Build history of the part. All positions in model axes, mm. A direction names the side the tool comes from. Coordinates: 2 decimals unless noted, no trailing zeros. Write each loop counter-clockwise with the first axis right and the second up, starting at its lowest first coordinate (ties: lowest second). Pieces come first, ordered by that corner, then holes. Notation, with made-up numbers: (88, 24) -> (141, 24) arc R33 cw to (141, 62) -> close; hole circle Ø10 at (5, -1). An arc over 180 degrees is marked (long way). Write each question's results on one line, items separated by ' | '. Start each with the question number.
Q1. Saw through at B-B on z = 32.5. Give the cut face in (x, y), and give its area (3 significant figures).
Q2. Tool access for faces 4 (the face through (6, 4, 26.303)), 5 (the face through (40, 5, -23.097)), 6 (the face through (-7.56, 11.65, -4.66)): list every direction of +Z, -Z, +X, -X, +Y, -Y with a clear straight run to the whole face (end or side of a thin tool).
Q3. Saw through at C-C on x = -15.5. Give the cut face in (y, z), and give its area (3 significant figures).
Q4. Saw through at A-A on z = 15.5. Give the cut face in (x, y), and give its area (3 significant figures).
Q5. Saw through at D-D on y = 13. Give the cut face in (x, z) (3 decimals), and give its area (3 significant figures).
Q6. Drop flat-ended pins along their axis: pin 1 Ø1 at (x, z) = (18, -14) entering from +Y; pin 2 Ø1 at (x, z) = (13, 28) entering from +Y; pin 3 Ø1.3 at (x, y) = (-6, 9) entering from -Z; pin 4 Ø5 at (y, z) = (9, -2) entering from -X. Give the stop position or say it passes through.
Q7. Drill centre lines: line 1 (X direction, y = 3, z = 11); line 2 (Y direction, x = 69, z = -8.5); line 3 (Y direction, x = 6.5, z = 4.5). Where is each one in solid material? Low to high.
Q8. Two-plate mould, pull along Z, no slides. Class faces 1 (the face through (-7, 15, 24)), 2 (the face through (4.412, 8, 29)), 3 (the face through (107.31, 5.03, -22.24)): released by +Z, released by -Z, zero draft, split by the parting line, or undercut.
from build123d import *

# Parameters (mm, degrees)
SKETCH1_W           = 134
SKETCH1_H           = 67
BOSS_EXTRUDE1_DEPTH = 10
SKETCH2_W           = 19.1
SKETCH2_H           = 19.1
CUT_EXTRUDE1_DEPTH  = 10
SKETCH2_3_R         = 1.275
BOSS_EXTRUDE2_DEPTH = 5
CUT_EXTRUDE3_START  = -1.6
SKETCH2_6_R         = 1.275
CUT_EXTRUDE3_DEPTH  = 1.6
SKETCH2_5_W         = 3.9
SKETCH2_5_H         = 3.1
SKETCH2_5_H_2       = 0.9
CUT_EXTRUDE2_DEPTH  = 3.14
FILLET1_R           = 3
FILLET2_R           = 1.5
FILLET3_R           = 1.5


with BuildPart() as part:
    # Sketch1 → Boss-Extrude1 (new body)
    with BuildSketch(Plane(origin=(0, 0, 0), x_dir=(1, 0, 0), z_dir=(0, 1, 0))):
        with Locations((41.212068984, -10.4030388)):
            Rectangle(SKETCH1_W, SKETCH1_H)
    extrude(amount=BOSS_EXTRUDE1_DEPTH)

    # Sketch2 → Cut-Extrude1 (cut)
    with BuildSketch(Plane(origin=(0, 10, 0), x_dir=(1, 0, 0), z_dir=(0, 1, 0))):
        with Locations((6.362068984, -16.7530388)):
            Rectangle(SKETCH2_W, SKETCH2_H)
    extrude(amount=-CUT_EXTRUDE1_DEPTH, mode=Mode.SUBTRACT)

    # Sketch2<3> → Boss-Extrude2 (add)
    with BuildSketch(Plane(origin=(0, 10, 0), x_dir=(1, 0, 0), z_dir=(0, 1, 0))):
        with Locations(Location((-6.787931016, 3.6469612, 0), (0, 0, 270))):
            Circle(SKETCH2_3_R)
        with Locations(Location((-6.787931016, -24.4530388, 0), (0, 0, 270))):
            Circle(SKETCH2_3_R)
        with Locations(Location((21.212068984, -24.4530388, 0), (0, 0, 270))):
            Circle(SKETCH2_3_R)
        with Locations(Location((21.212068984, 3.6469612, 0), (0, 0, 270))):
            Circle(SKETCH2_3_R)
    extrude(amount=BOSS_EXTRUDE2_DEPTH)

    # Sketch2<6> → Cut-Extrude3 (cut)
    with BuildSketch(Plane(origin=(0, 10, 0), x_dir=(1, 0, 0), z_dir=(0, 1, 0)).offset(CUT_EXTRUDE3_START)):
        Polygon((26.212068984, 8.5969612), (-11.787931016, 8.5969612), (-11.787931016, -29.4030388), (4.412068984, -29.4030388), (4.412068984, -26.3030388), (-3.187931016, -26.3030388), (-3.187931016, -7.2030388), (15.912068984, -7.2030388), (15.912068984, -26.3030388), (8.312068984, -26.3030388), (8.312068984, -29.4030388), (26.212068984, -29.4030388), align=None)
        with Locations(Location((-6.787931016, -24.4530388, 0), (0, 0, 270))):
            Circle(SKETCH2_6_R, mode=Mode.SUBTRACT)
        with Locations(Location((21.212068984, -24.4530388, 0), (0, 0, 270))):
            Circle(SKETCH2_6_R, mode=Mode.SUBTRACT)
        with Locations(Location((-6.787931016, 3.6469612, 0), (0, 0, 270))):
            Circle(SKETCH2_6_R, mode=Mode.SUBTRACT)
        with Locations(Location((21.212068984, 3.6469612, 0), (0, 0, 270))):
            Circle(SKETCH2_6_R, mode=Mode.SUBTRACT)
    extrude(amount=CUT_EXTRUDE3_DEPTH, mode=Mode.SUBTRACT)

    # Sketch2<5> → Cut-Extrude2 (cut)
    with BuildSketch(Plane(origin=(0, 10, 0), x_dir=(1, 0, 0), z_dir=(0, 1, 0))):
        with Locations((6.362068984, -27.8530388)):
            Rectangle(SKETCH2_5_W, SKETCH2_5_H)
        with Locations((6.362068984, -29.8530388)):
            Rectangle(SKETCH2_5_W, SKETCH2_5_H_2)
    extrude(amount=-CUT_EXTRUDE2_DEPTH, mode=Mode.SUBTRACT)

    # Fillet1
    fillet1_edges = [part.edges().sort_by_distance(p)[0] for p in [
        (108.212068984, 10, 10.4030388),
        (41.212068984, 10, -23.0969612),
        (-25.787931016, 10, 10.4030388),
        (41.212068984, 0, -23.0969612),
        (108.212068984, 0, 10.4030388),
        (41.212068984, 0, 43.9030388),
        (-25.787931016, 0, 10.4030388),
        (-25.787931016, 5, -23.0969612),
        (108.212068984, 5, -23.0969612),
        (108.212068984, 5, 43.9030388),
        (-25.787931016, 5, 43.9030388),
        (41.212068984, 10, 43.9030388),
    ]]
    fillet(fillet1_edges, radius=FILLET1_R)

    # Fillet2
    fillet2_edges = [part.edges().sort_by_distance(p)[0] for p in [
        (4.412068984, 7.63, 26.3030388),
        (6.362068984, 6.86, 26.3030388),
        (-3.187931016, 4.2, 26.3030388),
        (15.912068984, 4.2, 26.3030388),
        (15.912068984, 0, 16.7530388),
        (6.362068984, 0, 26.3030388),
        (-3.187931016, 0, 16.7530388),
        (15.912068984, 8.4, 16.7530388),
        (6.362068984, 8.4, 7.2030388),
        (12.112068984, 8.4, 26.3030388),
        (-3.187931016, 8.4, 16.7530388),
        (0.612068984, 8.4, 26.3030388),
        (8.312068984, 7.63, 26.3030388),
    ]]
    fillet(fillet2_edges, radius=FILLET2_R)

    # Fillet3
    fillet3_edges = [part.edges().sort_by_distance(p)[0] for p in [
        (7.212068984, 10, -8.5969612),
        (26.212068984, 10, 10.4030388),
        (-11.787931016, 10, 10.4030388),
    ]]
    fillet(fillet3_edges, radius=FILLET3_R)


solid = part.part
Returned:
1) outline: (-25.79, 3) arc R3 ccw to (-22.79, 0) -> (105.21, 0) arc R3 ccw to (108.21, 3) -> (108.21, 7) arc R3 ccw to (105.21, 10) -> (-22.79, 10) arc R3 ccw to (-25.79, 7) -> close | area: 1,330 mm2
2) face 4: +Y, -Y | face 5: -Z, +X, -X, +Y, -Y | face 6: +Y
3) outline: (0, -20.1) arc R3 ccw to (3, -23.1) -> (7, -23.1) arc R3 ccw to (10, -20.1) -> (10, 40.9) arc R3 ccw to (7, 43.9) -> (3, 43.9) arc R3 ccw to (0, 40.9) -> close | area: 662 mm2
4) outline: (-25.79, 3) arc R3 ccw to (-22.79, 0) -> (-4.69, 0) arc R1.5 ccw to (-3.19, 1.5) -> (-3.19, 6.9) arc R1.5 ccw to (-4.69, 8.4) -> (-11.79, 8.4) -> (-11.79, 8.5) arc R1.5 ccw to (-13.29, 10) -> (-22.79, 10) arc R3 ccw to (-25.79, 7) -> close; (15.91, 1.5) arc R1.5 ccw to (17.41, 0) -> (105.21, 0) arc R3 ccw to (108.21, 3) -> (108.21, 7) arc R3 ccw to (105.21, 10) -> (27.71, 10) arc R1.5 ccw to (26.21, 8.5) -> (26.21, 8.4) -> (17.41, 8.4) arc R1.5 ccw to (15.91, 6.9) -> close | area: 1,110 mm2
5) outline: circle Ø2.55 at (-6.788, -3.647); circle Ø2.55 at (-6.788, 24.453); circle Ø2.55 at (21.212, -3.647); circle Ø2.55 at (21.212, 24.453) | area: 20.4 mm2
6) pin 1: stops at y = 10 | pin 2: stops at y = 8.4 | pin 3: stops at z = -22.78 | pin 4: stops at x = -25.79
7) line 1: x = -25.79 to -3.19, 15.91 to 108.21 | line 2: y = 0 to 10 | line 3: y = 0 to 8.4
8) face 1: zero draft | face 2: undercut | face 3: released by -Z
